Geometry: final body of the model. Coordinates: model frame, mm. A direction names the side the tool comes from. Give positions to 0.01 mm unless a question says otherwise; leave off trailing zeros.
Autodesk Inventor part; units mm, degrees
ref_plane "YZ Plane" through (0, 0, 0) normal (1, 0, 0) x (0, 1, 0)
ref_plane "XZ Plane" through (0, 0, 0) normal (0, 1, 0) x (-1, 0, 0)
ref_plane "XY Plane" through (0, 0, 0) normal (0, 0, 1) x (1, 0, 0)
sketch "Sketch1" plane through (0, 0, 0) normal (0, 1, 0) x (-1, 0, 0)
  circle A0 centre (0, 0) radius 15
  line L0 (0, -25) -> (10.866, -25)
  line L1 (0, -25) -> (-10.866, -25)
  line L2 (-10.866, -25) -> (0, -43.8205)
  line L3 (0, -43.8205) -> (10.866, -25)
  circle A1 centre (0, 0) radius 16.5
  line L4 (13.4641, -23.5) -> (0, -23.5)
  line L5 (0, -23.5) -> (-13.4641, -23.5)
  line L6 (-13.4641, -23.5) -> (0, -46.8205)
  line L7 (0, -46.8205) -> (13.4641, -23.5)
  line L8 (25, 0) -> (25, 10.866)
  line L9 (25, 0) -> (25, -10.866)
  line L10 (25, -10.866) -> (43.8205, 0)
  line L11 (43.8205, 0) -> (25, 10.866)
  line L12 (23.5, 13.4641) -> (23.5, 0)
  line L13 (23.5, 0) -> (23.5, -13.4641)
  line L14 (23.5, -13.4641) -> (46.8205, 0)
  line L15 (46.8205, 0) -> (23.5, 13.4641)
  line L16 (0, 25) -> (-10.866, 25)
  line L17 (0, 25) -> (10.866, 25)
  line L18 (10.866, 25) -> (0, 43.8205)
  line L19 (0, 43.8205) -> (-10.866, 25)
  line L20 (-13.4641, 23.5) -> (0, 23.5)
  line L21 (0, 23.5) -> (13.4641, 23.5)
  line L22 (13.4641, 23.5) -> (0, 46.8205)
  line L23 (0, 46.8205) -> (-13.4641, 23.5)
  line L24 (-25, 0) -> (-25, -10.866)
  line L25 (-25, 0) -> (-25, 10.866)
  line L26 (-25, 10.866) -> (-43.8205, 0)
  line L27 (-43.8205, 0) -> (-25, -10.866)
  line L28 (-23.5, -13.4641) -> (-23.5, 0)
  line L29 (-23.5, 0) -> (-23.5, 13.4641)
  line L30 (-23.5, 13.4641) -> (-46.8205, 0)
  line L31 (-46.8205, 0) -> (-23.5, -13.4641)
  line L32 (46.8205, 46.8205) -> (25.8205, 46.8205)
  line L33 (25.8205, 46.8205) -> (25.8205, 20.8205)
  line L34 (25.8205, 20.8205) -> (46.8205, 20.8205)
  line L35 (46.8205, 20.8205) -> (46.8205, 46.8205)
  line L36 (46.8205, -46.8205) -> (25.8205, -46.8205)
  line L37 (25.8205, -46.8205) -> (25.8205, -20.8205)
  line L38 (25.8205, -20.8205) -> (46.8205, -20.8205)
  line L39 (46.8205, -20.8205) -> (46.8205, -46.8205)
  line L40 (27.3205, 22.3205) -> (27.3205, 45.3205)
  line L41 (27.3205, 45.3205) -> (45.3205, 45.3205)
  line L42 (45.3205, 45.3205) -> (45.3205, 22.3205)
  line L43 (45.3205, 22.3205) -> (27.3205, 22.3205)
  line L44 (45.3205, -45.3205) -> (27.3205, -45.3205)
  line L45 (27.3205, -45.3205) -> (27.3205, -22.3205)
  line L46 (27.3205, -22.3205) -> (45.3205, -22.3205)
  line L47 (45.3205, -22.3205) -> (45.3205, -45.3205)
  line L48 (0, 60) -> (60, 60)
  line L49 (60, 60) -> (60, -60)
  line L50 (60, -60) -> (-60, -60)
  line L51 (-60, -60) -> (-60, 60)
  line L52 (-60, 60) -> (0, 60)
  dimension "d0" = 30
  dimension "d5" = 33
  dimension "d6" = 1.5
  dimension "d10" = 360
  dimension "d12" = 21
  dimension "d13" = 26
  dimension "d14" = 21
  dimension "d15" = 26
  dimension "d16" = 1.5
  dimension "d17" = 1.5
  dimension "d18" = 60
  dimension "d19" = 120
  dimension "d20" = 120
  dimension "d21" = 120
extrude "Extrusion1" add sketch "Sketch1" along normal blind 20 contours L48 L49 L50 L51 L52
sketch "Sketch2" plane through (0, 20, 0) normal (0, 1, 0) x (1, 0, 0)
  line L0 (-49.5, -21) -> (-49.5, -49.3205)
  line L1 (-49.5, -49.3205) -> (-23.5, -49.3205)
  line L2 (-23.5, -49.3205) -> (-23.5, -18.3205)
  line L3 (-23.5, -18.3205) -> (-49.5, -18.3205)
  line L4 (-49.5, -18.3205) -> (-49.5, -49.3205)
  line L5 (-49.5, 21) -> (-49.5, 49.3205)
  line L6 (-49.5, 49.3205) -> (-23.5, 49.3205)
  line L7 (-23.5, 49.3205) -> (-23.5, 18.3205)
  line L8 (-23.5, 18.3205) -> (-49.5, 18.3205)
  line L9 (-49.5, 18.3205) -> (-49.5, 49.3205)
  line L10 (-21, 0) -> (-21, 17.7942)
  line L11 (-51.8205, 0) -> (-21, 17.7942)
  line L12 (-21, -17.7942) -> (-51.8205, 0)
  line L13 (-21, 0) -> (-21, -17.7942)
  line L14 (0, -21) -> (-17.7942, -21)
  line L15 (0, -51.8205) -> (-17.7942, -21)
  line L16 (17.7942, -21) -> (0, -51.8205)
  line L17 (0, -21) -> (17.7942, -21)
  line L18 (21, 0) -> (21, -17.7942)
  line L19 (51.8205, 0) -> (21, -17.7942)
  line L20 (21, 17.7942) -> (51.8205, 0)
  line L21 (21, 0) -> (21, 17.7942)
  line L22 (0, 21) -> (17.7942, 21)
  line L23 (0, 51.8205) -> (17.7942, 21)
  line L24 (-17.7942, 21) -> (0, 51.8205)
  line L25 (0, 21) -> (-17.7942, 21)
  circle A0 centre (0, 0) radius 19
  point P0 (-25.8205, -46.8205)
  point P1 (-25.8205, 46.8205)
  dimension "d34" = 360
extrude "Extrusion2" cut sketch "Sketch2" against normal blind 4
fillet "Fillet1" radius 5 4 edges at (-60, 10, -60) (60, 10, -60) (60, 10, 60) (-60, 10, 60)
fillet "Fillet2" radius 5 8 edges at (-58.5355, 0, 58.5355) (-60, 0, 0) (-58.5355, 0, -58.5355) (0, 0, -60) (58.5355, 0, -58.5355) (60, 0, 0) (58.5355, 0, 58.5355) (0, 0, 60)
fillet "Fillet3" radius 2 21 edges at (-35.1603, 0, 6.7321) (-35.1603, 0, -6.7321) (-23.5, 0, 0) (-25.8205, 0, -33.8205) (-36.3205, 0, -20.8205) (-46.8205, 0, -33.8205) (-36.3205, 0, -46.8205) (6.7321, 0, -35.1603) (-6.7321, 0, -35.1603) (0, 0, -23.5) (35.1603, 0, -6.7321) (23.5, 0, 0) (35.1603, 0, 6.7321) (16.5, 0, 0) (0, 0, 23.5) (6.7321, 0, 35.1603) (-6.7321, 0, 35.1603) (-25.8205, 0, 33.8205) (-36.3205, 0, 20.8205) (-46.8205, 0, 33.8205) (-36.3205, 0, 46.8205)
fillet "Fillet4" radius 5 8 edges at (-58.5355, 20, 58.5355) (0, 20, 60) (58.5355, 20, 58.5355) (60, 20, 0) (58.5355, 20, -58.5355) (0, 20, -60) (-58.5355, 20, -58.5355) (-60, 20, 0)
fillet "Fillet5" radius 1 18 edges at (16.5, 16, 0) (-25.8205, 16, 33.8205) (-36.3205, 16, 46.8205) (-46.8205, 16, 33.8205) (-36.3205, 16, 20.8205) (-36.3205, 16, -20.8205) (-46.8205, 16, -33.8205) (-25.8205, 16, -33.8205) (-36.3205, 16, -46.8205) (0, 16, -23.5) (-6.7321, 16, -35.1603) (6.7321, 16, -35.1603) (6.7321, 16, 35.1603) (-6.7321, 16, 35.1603) (0, 16, 23.5) (35.1603, 16, 6.7321) (23.5, 16, 0) (35.1603, 16, -6.7321)
properties part number "Vo_Nut_Bam" material "Water"
Item 1: Ray query, probe 1 along X at (y, z) = (7.5, 0); probe 2 along X at (y, z) = (19, 0); probe 3 along Z at (x, y) = (-30.5, 12.25). Return the intervals inside material, ascending.
Values follow:
probe 1: x = -60 to -46.82, -23.5 to -16.5, 16.5 to 23.5, 46.82 to 60
probe 2: x = -58 to -51.82, -21 to -19, 19 to 21, 51.82 to 58
probe 3: z = -60 to -46.82, -20.82 to -9.42, 9.42 to 20.82, 46.82 to 60
Item 2: Draft query along Z for faces 1 (the face through (-60, 10, 1)), 2 (the face through (58, 10, 59)), 3 (the face through (-34.997, 8.902, -6.826)). Return one class per face: +Z half, -Z half, draft (parallel to the pull), parting line (faces both ways), or undercut.
Values follow:
face 1: draft
face 2: +Z half
face 3: undercut
Item 3: Pin query (flat end, axial travel): pin 1 (1.2 mm diameter, centred on x = -30.5, y = 18, fed in from -Z); pin 2 (4.5 mm diameter, centred on x = 5.5, y = 17.5, fed in from +Z); pin 3 (9 mm diameter, centred on x = -31, z = 5.5, fed in from +Y); pin 4 (3 mm diameter, centred on x = -27.5, z = 37, fed in from +Y). Return the tip coordinate at first contact, or that it passes through.
Values follow:
pin 1: stops at z = -59.39
pin 2: stops at z = 59.99
pin 3: stops at y = 16
pin 4: passes through
Item 4: Section query A-A on y = 12.5. Give the number of separate pieces and of enclosed holes in the cut face, plus the area to 3 significant figures.
Values follow:
separate pieces: 1
enclosed holes: 7
area: 11,200 mm2
Item 5: Set-up query: faces 4 (the face through (-8, 16, -35.3)), 5 (the face through (-23.5, 9, 0)), 6 (the face through (25, 20, 25)). Return all of +Z, -Z, +X, -X, +Y, -Y with unobstructed straight access to the full face (end or side cutting, diameter ignored); none if empty.
Values follow:
face 4: +Y
face 5: +Y, -Y
face 6: +Z, -Z, +X, -X, +Y
